Geometry: final body of the model. Coordinates: model frame, mm. Face numbers are marked on the shaded views. Coordinates: 2 decimals unless noted, no trailing zeros. Loops run counter-clockwise (first coordinate to the right, second up) from the corner with the lowest first, then second, coordinate; pieces in that order, holes last. Notation, with made-up numbers: (-21.75, 64.5) -> (34.25, 64.5) arc R13 ccw to (34.25, 76.5) -> close; hole circle Ø10 at (88.25, -26). An arc over 180 degrees is marked (long way). One line per item, written item: value. Start each with the question number.
from build123d import *

# Parameters (mm, degrees)
SKETCH1_W            = 17.902420718
SKETCH1_H            = 25.880604579
BOSS_EXTRUDE1_DEPTH  = 6
LPATTERN1_COUNT      = 3
LPATTERN1_PITCH      = 8
LPATTERN1_COUNT_DIR2 = 2
LPATTERN1_PITCH_DIR2 = 8


with BuildPart() as part:
    # Sketch1 → Boss-Extrude1 (new body)
    with BuildSketch(Plane(origin=(0, 0, 0), x_dir=(1, 0, 0), z_dir=(0, 1, 0))):
        with Locations((3.951210359, 12.940302289)):
            Rectangle(SKETCH1_W, SKETCH1_H)
    extrude(amount=BOSS_EXTRUDE1_DEPTH)

    # Sketch3 → Cut-Revolve1 (revolve, cut)
    with BuildSketch(Plane.ZY, mode=Mode.PRIVATE) as cut_revolve1_sk:
        Polygon((-5, 6), (-5, 0), (-6.77, 0), (-6.77, 3.2), (-6.965795073, 6), align=None)
    cut_revolve1 = revolve(cut_revolve1_sk.sketch.rotate(Axis((0, 6, -5), (0, -1, 0)), 180), axis=Axis((0, 6, -5), (0, -1, 0)), mode=Mode.SUBTRACT)

    # LPattern1: Cut-Revolve1 3 × 2
    with Locations(*[(j * LPATTERN1_PITCH_DIR2, 0, -i * LPATTERN1_PITCH) for i in range(LPATTERN1_COUNT) for j in range(LPATTERN1_COUNT_DIR2) if (i, j) != (0, 0)]):
        add(cut_revolve1, mode=Mode.SUBTRACT)


solid = part.part
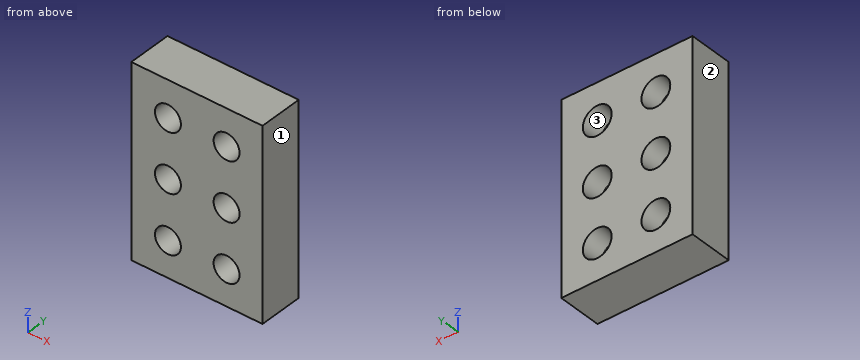
1. Line query: L1, parallel to X at y = 2.05, z = -21; L2, parallel to Z at x = 8, y = 2.5; L3, parallel to Z at x = -1.5, y = 0.4. Output: solid intervals per line, ascending. Write a range as [from, to].
2. Draft query along X for the marked faces 1, 2 and 3. Return one class per face: released by +X, released by -X, zero draft, split by the parting line, or undercut.
3. Section D-D on y = 4.75. Return the cut outline in (x, z).
4. Section B-B on z = -21. Return the cut outline in (x, y).
5. Section C-C on x = 9.5. Count the separate pieces of the cut face and the enclosed holes in it, plus the area to 3 significant figures.
6. Section A-A on y = 2.75. Return the cut outline in (x, z).
Checks:
1. L1: [-5, -1.77], [1.77, 6.23], [9.77, 12.9]
1. L2: [-25.88, -22.77], [-19.23, -14.77], [-11.23, -6.77], [-3.23, 0]
1. L3: [-25.88, -21.94], [-20.06, -13.94], [-12.06, -5.94], [-4.06, 0]
2. face 1: released by +X
2. face 2: released by -X
2. face 3: undercut
3. outline: (-5, -25.88) -> (12.9, -25.88) -> (12.9, 0) -> (-5, 0) -> close; hole circle Ø3.76 at (0, -21); hole circle Ø3.76 at (0, -13); hole circle Ø3.76 at (0, -5); hole circle Ø3.76 at (8, -21); hole circle Ø3.76 at (8, -13); hole circle Ø3.76 at (8, -5)
4. outline: (-5, 0) -> (-1.77, 0) -> (-1.77, 3.2) -> (-1.97, 6) -> (-5, 6) -> close; (1.77, 0) -> (6.23, 0) -> (6.23, 3.2) -> (6.03, 6) -> (1.97, 6) -> (1.77, 3.2) -> close; (9.77, 0) -> (12.9, 0) -> (12.9, 6) -> (9.97, 6) -> (9.77, 3.2) -> close
5. separate pieces: 4
5. enclosed holes: 0
5. area: 119 mm²
6. outline: (-5, -25.88) -> (12.9, -25.88) -> (12.9, 0) -> (-5, 0) -> close; hole circle Ø3.54 at (0, -21); hole circle Ø3.54 at (0, -13); hole circle Ø3.54 at (0, -5); hole circle Ø3.54 at (8, -21); hole circle Ø3.54 at (8, -13); hole circle Ø3.54 at (8, -5)
